Can you work these out from the model? Positions are in its coordinate system, mm. Face numbers are marked on the shaded views. A direction names the side the tool comes from. Round coordinates to 2 decimals unless told otherwise and drop trailing zeros. Loops run counter-clockwise (first coordinate to the right, second up) from the corner with the lowest first, then second, coordinate; pieces in that order, holes last.
from build123d import *

# Parameters (mm, degrees)
SKETCH1_W                = 90
SKETCH1_H                = 20
BOSS_EXTRUDE1_DEPTH      = 60
SKETCH2_W                = 40
SKETCH2_H                = 10
CUT_EXTRUDE2_DEPTH       = 90
SKETCH3_W                = 15
SKETCH3_H                = 12.908253666
CUT_EXTRUDE4_DEPTH       = 30
BOSS_EXTRUDE7_DEPTH      = 10
BOSS_EXTRUDE7_DEPTH_BACK = 60
SKETCH4_W                = 15
SKETCH4_H                = 50.029295458
CUT_EXTRUDE7_DEPTH       = 15
SKETCH15_R               = 13
BOSS_EXTRUDE9_DEPTH      = 30
SKETCH28_W               = 15
SKETCH28_H               = 31.312087749
BOSS_EXTRUDE12_DEPTH     = 47
CUT_EXTRUDE10_DEPTH      = 15


with BuildPart() as part:
    # Sketch1 → Boss-Extrude1 (new body)
    with BuildSketch(Plane.XY):
        with Locations((5.654450262, 10)):
            Rectangle(SKETCH1_W, SKETCH1_H)
    extrude(amount=BOSS_EXTRUDE1_DEPTH)

    # Sketch2 → Cut-Extrude2 (cut)
    with BuildSketch(Plane(origin=(50.654450262, 0, 0), x_dir=(0, 0, -1), z_dir=(1, 0, 0))):
        with Locations((-30, 5)):
            Rectangle(SKETCH2_W, SKETCH2_H)
    extrude(amount=-CUT_EXTRUDE2_DEPTH, mode=Mode.SUBTRACT)

    # Sketch3 → Cut-Extrude4 (cut)
    with BuildSketch(Plane(origin=(0, 20, 0), x_dir=(1, 0, 0), z_dir=(0, 1, 0))):
        with Locations((-19.345549738, -30)):
            Rectangle(SKETCH3_W, SKETCH3_H)
        with Locations((30.654450262, -30)):
            Rectangle(SKETCH3_W, SKETCH3_H)
    extrude(amount=-CUT_EXTRUDE4_DEPTH, mode=Mode.SUBTRACT)

    # Sketch4 → Boss-Extrude7 (add, two sides: drawn at the far end of the back side and taken through both)
    with BuildSketch(Plane(origin=(0, 0, 0), x_dir=(-1, 0, 0), z_dir=(0, 0, -1)).offset(-BOSS_EXTRUDE7_DEPTH_BACK)):
        with Locations((-5.654450262, 45.014647729)):
            Rectangle(SKETCH4_W, SKETCH4_H)
    extrude(amount=BOSS_EXTRUDE7_DEPTH + BOSS_EXTRUDE7_DEPTH_BACK)

    # Sketch13 → Cut-Extrude7 (cut)
    with BuildSketch(Plane.ZY.offset(1.845549738)):
        Polygon((60, 20), (60, 70.029295458), (0, 70.029295458), align=None)
    extrude(amount=-CUT_EXTRUDE7_DEPTH, mode=Mode.SUBTRACT)

    # Sketch15 → Boss-Extrude9 (add)
    with BuildSketch(Plane(origin=(0, 70.029295458, 0), x_dir=(1, 0, 0), z_dir=(0, 1, 0))):
        with BuildLine():
            Line((-1.845549738, 10), (13.154450262, 10))
            Line((13.154450262, 10), (13.154450262, 31.312087749))
            ThreePointArc((13.154450262, 31.312087749), (5.654450262, 70.136734201), (-1.845549738, 31.312087749))
            Line((-1.845549738, 31.312087749), (-1.845549738, 10))
        make_face()
        with Locations(Location((5.654450262, 50, 0), (0, 0, 270))):
            Circle(SKETCH15_R, mode=Mode.SUBTRACT)
    extrude(amount=-BOSS_EXTRUDE9_DEPTH)

    # Sketch28 → Boss-Extrude12 (add)
    with BuildSketch(Plane.XZ):
        with Locations((5.654450262, -15.656043875)):
            Rectangle(SKETCH28_W, SKETCH28_H)
    extrude(amount=-BOSS_EXTRUDE12_DEPTH)

    # Sketch29 → Cut-Extrude10 (cut)
    with BuildSketch(Plane(origin=(13.154450262, 0, 0), x_dir=(0, 0, -1), z_dir=(1, 0, 0))):
        Polygon((31.312087749, 40.029295458), (0, 0), (31.312087749, 0), align=None)
    extrude(amount=-CUT_EXTRUDE10_DEPTH, mode=Mode.SUBTRACT)


solid = part.part
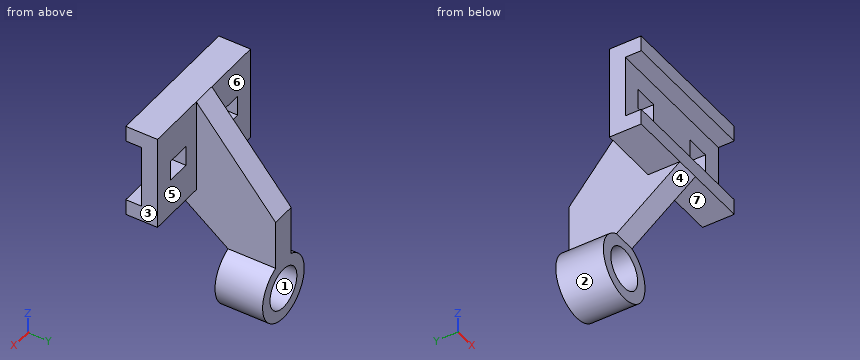
(1) Will these pins go through, and if not, where does the flat tip stop? P1, Ø10, axis at x = 24.5, y = 9.5, coming from the -Z side; P2, Ø4, axis at x = -9.5, y = 43.5, coming from the +Z side; P3, Ø11, axis at x = -27.5, z = 22.5, coming from the +Y side; P4, Ø1.5, axis at x = -8, z = 9, coming from the -Y side.
Worked answers:
P1: stops at z = 0
P2: stops at z = -34.75
P3: stops at y = 20
P4: stops at y = 0
(2) If we section it at B-B, the plane x = -20: List the corners of the cut face in (y, z) for me, then the cut area to 3 significant figures.
Worked answers:
outline: (0, 0) - (20, 0) - (20, 23.55) - (10, 23.55) - (10, 10) - (0, 10) - close; (0, 50) - (10, 50) - (10, 36.45) - (20, 36.45) - (20, 60) - (0, 60) - close
area: 671 mm2
(3) If we section it at A-A, the plane z = -50: List the corners of the cut face in (x, y) for me.
Worked answers:
outline: (-14.48, 40.03) - (-7.35, 40.03) - (-7.35, 70.03) - (-14.48, 70.03) - close; (18.65, 40.03) - (25.79, 40.03) - (25.79, 70.03) - (18.65, 70.03) - close
(4) For the marked faces 5, 6 and 7, which set-ups out of +Z, -Z, +X, -X, +Y, -Y let a thin tool reach every point of the face, with its end or its side?
Worked answers:
face 5: +Z, -Z, +X, +Y
face 6: +Z, -Z, -X, +Y
face 7: -Z, +X, +Y, -Y
(5) If I drill on line 1 (X direction, y = 55.75, z = -50); line 2 (Z direction, x = -26.5, y = 7.5); line 3 (Z direction, x = -9.5, y = 15), over which ranges is the centre line in solid material (lowest first)?
Worked answers:
line 1: x = -14.48 to -7.35, 18.65 to 25.79
line 2: z = 0 to 10, 50 to 60
line 3: z = 0 to 60
(6) If we section it at C-C, the plane y = 63.5: List the corners of the cut face in (x, z) for me, then the cut area to 3 significant figures.
Worked answers:
outline: (-1.85, -31.31) arc R20.14 ccw (long way) to (13.15, -31.31) - (13.15, 7.83) - (-1.85, 7.83) - close; hole circle Ø26 at (5.65, -50)
area: 1,320 mm2
(7) If we mould it in two halves opening along X, with no side actions, what happens to the marked faces 1, 2, 3 and 4? For each: released by +X, released by -X, zero draft, split by the parting line, or undercut.
Worked answers:
face 1: undercut
face 2: split by the parting line
face 3: released by +X
face 4: zero draft
(8) If we section it at D-D, the plane x = 11.5: List the corners of the cut face in (y, z) for me, then the cut area to 3 significant figures.
Worked answers:
outline: (0, 0) - (40.03, -31.31) - (40.03, -38.39) - (70.03, -38.39) - (70.03, 0) - (20, 60) - (0, 60) - (0, 50) - (10, 50) - (10, 10) - (0, 10) - close; (40.03, -69.27) - (70.03, -69.27) - (70.03, -61.61) - (40.03, -61.61) - close
area: 4,310 mm2
